The model under review builds one solid part; all positions refer to its coordinate system, in mm. A direction names the side the tool comes from. Round coordinates to 2 decimals unless told otherwise and drop trailing zeros. Order: outer loops, then holes, each group sorted by start corner. A loop starts at its lowest first (then second) coordinate and runs counter-clockwise, first axis right, second up.
```python
from build123d import *

# Parameters (mm, degrees)
F1_DEPTH = 152.4
F2_DEPTH = 31.75
F3_W     = 73.3992542744
F3_H     = 43.9409847975
F3_W_2   = 60.6992542744
F3_H_2   = 31.2409847975
F4_DEPTH = 6.35
F5_SIZE  = 2.54
F6_R     = 19.05
F6_R_2   = 12.7
F7_DEPTH = 12.7


# Not quite as in the source:
# - a feature names something its author has since deleted; it is built from what else it names


with BuildPart() as f1:
    # F0 (on Top) → F1 (new body)
    with BuildSketch(Plane.XY):
        with BuildLine():
            Line((0, 228.6), (0, 44.45))
            ThreePointArc((0, 44.45), (31.4308964237, 31.4308964237), (44.45, 0))
            ThreePointArc((44.45, 0), (31.4308964237, -31.4308964237), (0, -44.45))
            Line((0, -44.45), (0, -139.7))
            Line((0, -139.7), (114.3, -139.7))
            Line((114.3, -139.7), (114.3, 228.6))
            Line((114.3, 228.6), (0, 228.6))
        make_face()
        with BuildLine():
            ThreePointArc((0, -44.45), (-44.45, 0), (0, 44.45))
            Line((0, 44.45), (0, 228.6))
            Line((0, 228.6), (-114.3, 228.6))
            Line((-114.3, 228.6), (-114.3, -139.7))
            Line((-114.3, -139.7), (0, -139.7))
            Line((0, -139.7), (0, -44.45))
        make_face()
        with BuildLine():
            Line((0, 44.45), (0, 0))
            Line((0, 0), (0, -44.45))
            ThreePointArc((0, -44.45), (31.4308964237, -31.4308964237), (44.45, 0))
            ThreePointArc((44.45, 0), (31.4308964237, 31.4308964237), (0, 44.45))
        make_face()
        with BuildLine():
            Line((0, -44.45), (0, 0))
            Line((0, 0), (0, 44.45))
            ThreePointArc((0, 44.45), (-44.45, 0), (0, -44.45))
        make_face()
    extrude(amount=F1_DEPTH)

    # F0 (on Top) → F2 (join)
    with BuildSketch(Plane.XY):
        with BuildLine():
            Line((0, 44.45), (0, 0))
            Line((0, 0), (0, -44.45))
            ThreePointArc((0, -44.45), (31.4308964237, -31.4308964237), (44.45, 0))
            ThreePointArc((44.45, 0), (31.4308964237, 31.4308964237), (0, 44.45))
        make_face()
        with BuildLine():
            Line((0, -44.45), (0, 0))
            Line((0, 0), (0, 44.45))
            ThreePointArc((0, 44.45), (-44.45, 0), (0, -44.45))
        make_face()
    extrude(amount=-F2_DEPTH)

    # F3 (on face) → F4 (join)
    with BuildSketch(Plane(origin=(0, 228.6, 0), x_dir=(-1, 0, 0), z_dir=(0, 1, 0))):
        with Locations((58.9650124311, 110.7811406255)):
            Rectangle(F3_W, F3_H)
        with Locations((58.9650124311, 110.7811406255)):
            Rectangle(F3_W_2, F3_H_2, mode=Mode.SUBTRACT)
    extrude(amount=F4_DEPTH)

    # F5
    f5_edges = [f1.edges().sort_by_distance(p)[0] for p in [
        (-95.66464, 234.95, 110.781141),
        (-58.965012, 234.95, 88.810648),
        (-22.265385, 234.95, 110.781141),
        (-58.965012, 234.95, 132.751633),
    ]]
    chamfer(f5_edges, length=F5_SIZE)

    # F6 (on face) → F7 (join)
    with BuildSketch(Plane.XZ.offset(139.7)):
        with BuildLine():
            ThreePointArc((53.975, 57.15), (34.925, 76.2), (15.875, 57.15))
            ThreePointArc((15.875, 57.15), (34.925, 38.1), (53.975, 57.15))
        make_face()
        with BuildLine():
            ThreePointArc((47.625, 57.15), (34.925, 44.45), (22.225, 57.15))
            ThreePointArc((22.225, 57.15), (34.925, 69.85), (47.625, 57.15))
        make_face(mode=Mode.SUBTRACT)
        with Locations((-34.925, 57.15)):
            Circle(F6_R)
        with Locations((-34.925, 57.15)):
            Circle(F6_R_2, mode=Mode.SUBTRACT)
    extrude(amount=F7_DEPTH)


solid = f1.part
```
(1) To check wall thickness, follow probe 1 along Z at (x, y) = (62, 3); probe 2 along Y at (x, z) = (-24, 8.5); probe 3 along Y at (x, z) = (-2, -7.5). State the ranges of each line that lie inside material, in increasing order.
Data:
probe 1: z = 0 to 152.4
probe 2: y = -139.7 to 228.6
probe 3: y = -44.4 to 44.4
(2) Consider section C-C (z = 57.15). Write out the cut boundary in (x, y) (3 decimals), and give its area (3 significant figures).
Data:
outline: (-114.3, -139.7) - (-53.975, -139.7) - (-53.975, -152.4) - (-47.625, -152.4) - (-47.625, -139.7) - (-22.225, -139.7) - (-22.225, -152.4) - (-15.875, -152.4) - (-15.875, -139.7) - (15.875, -139.7) - (15.875, -152.4) - (22.225, -152.4) - (22.225, -139.7) - (47.625, -139.7) - (47.625, -152.4) - (53.975, -152.4) - (53.975, -139.7) - (114.3, -139.7) - (114.3, 228.6) - (-114.3, 228.6) - close
area: 84,500 mm2
(3) Insertion check: pin 1 (1.5 mm diameter, centred on x = -14.5, z = 46.5, fed in from +Y); pin 2 (3 mm diameter, centred on x = -65, y = 232, fed in from +Z); pin 3 (12 mm diameter, centred on x = 43, y = 162, fed in from -Z). Each pin has a flat end and moves straight along its axis. Give the tip position at first contact, or say it passes through.
Data:
pin 1: stops at y = 228.6
pin 2: stops at z = 132.75
pin 3: stops at z = 0
(4) Draft analysis for pull direction X (two halves, no side actions). For faces 1 (the cylindrical face through (37.678, -145.961, 44.752)), 2 (the cylindrical face through (-37.678, -145.961, 44.752)), 3 (the flat face through (114.3, 42, 75)), 4 (the flat face through (-54, 234.95, 95)), state which applies: pulls with the +X half, pulls with the -X half, needs draft (parallel to the pull), parting line crosses it, or undercut.
Data:
face 1: undercut
face 2: undercut
face 3: pulls with the +X half
face 4: needs draft
(5) Consider section D-D (y = -71.5). Write out the cut boundary in (x, z).
Data:
outline: (-114.3, 0) - (114.3, 0) - (114.3, 152.4) - (-114.3, 152.4) - close
(6) Consider section B-B (y = -26.5). Write out the cut boundary in (x, z), and give its area (3 significant figures).
Data:
outline: (-114.3, 0) - (-35.69, 0) - (-35.69, -31.75) - (35.69, -31.75) - (35.69, 0) - (114.3, 0) - (114.3, 152.4) - (-114.3, 152.4) - close
area: 37,100 mm2
(7) For faces 5 (the flat face through (-59, 228.6, 111)), 6 (the flat face through (-2, 47, 152.4)), 7 (the cylindrical face through (-48.97, -145.96, 70.02)), list the 3-axis set-ups (+Z, -Z, +X, -X, +Y, -Y) from which the entire face can be reached by the end or side of a thin tool; tool diameter is ignored.
Data:
face 5: +Y
face 6: +Z, +X, -X, +Y, -Y
face 7: -Y
(8) Consider section A-A (z = 121.5). Write out the cut boundary in (x, y), and give its area (3 significant figures).
Data:
outline: (-114.3, -139.7) - (114.3, -139.7) - (114.3, 228.6) - (-22.27, 228.6) - (-22.27, 232.41) - (-24.81, 234.95) - (-28.62, 234.95) - (-28.62, 228.6) - (-89.31, 228.6) - (-89.31, 234.95) - (-93.12, 234.95) - (-95.66, 232.41) - (-95.66, 228.6) - (-114.3, 228.6) - close
area: 84,300 mm2
